Build history of the part. All positions in model axes, mm. A direction names the side the tool comes from. Round coordinates to 2 decimals unless told otherwise and drop trailing zeros. Order: outer loops, then holes, each group sorted by start corner. A loop starts at its lowest first (then second) coordinate and runs counter-clockwise, first axis right, second up. Notation, with made-up numbers: M 14.25,30 L 66.25,30 A18 ccw 66.25,45 Z; hole C 55,-17 d7. An arc over 180 degrees is marked long. Use CSV: the item, a comma, the result in double quotes.
from build123d import *

# Parameters (mm, degrees)
SKETCH3_R           = 43
SKETCH3_R_2         = 41
BOSS_EXTRUDE1_DEPTH = 200


with BuildPart() as part:
    # Sketch3 → Boss-Extrude1 (new body)
    with BuildSketch(Plane(origin=(0, 0, 0), x_dir=(1, 0, 0), z_dir=(0, 1, 0))):
        with BuildLine():
            Line((15.84339478, 39.974827602), (33, 43))
            Line((33, 43), (33, 54.159072389))
            Line((33, 54.159072389), (31, 54.159072389))
            Line((31, 54.159072389), (31, 45))
            Line((31, 45), (-31, 45))
            Line((-31, 45), (-31, 54))
            Line((-31, 54), (-33, 54))
            Line((-33, 54), (-33, 43))
            Line((-33, 43), (-15.84339478, 39.974827602))
            ThreePointArc((-15.84339478, 39.974827602), (0, 43), (15.84339478, 39.974827602))
        make_face()
        Circle(SKETCH3_R)
        Circle(SKETCH3_R_2, mode=Mode.SUBTRACT)
    extrude(amount=BOSS_EXTRUDE1_DEPTH)


solid = part.part
(1) Tool access for faces 1 (the face through (-9, 99, 40)), 2 (the face through (-33, 99, -49)), 3 (the face through (16, 0, -38)), 4 (the face through (31, 99, -50)), 5 (the face through (33, 99, -49)): list every direction of +Z, -Z, +X, -X, +Y, -Y with a clear straight run to the whole face (end or side of a thin tool).
Answer block:
face 1,"+Y, -Y"
face 2,"-Z, -X, +Y, -Y"
face 3,"+Z, -Z, +X, -X, -Y"
face 4,"-Z, +Y, -Y"
face 5,"-Z, +X, +Y, -Y"
(2) Cut at D-D, the plane x = 25. Give the cut face in (y, z), and give its area (3 significant figures).
Answer block:
outline,"M 0,-45 L 200,-45 L 200,-41.59 L 0,-41.59 Z; M 0,-34.99 L 200,-34.99 L 200,-32.5 L 0,-32.5 Z; M 0,32.5 L 200,32.5 L 200,34.99 L 0,34.99 Z"
area,"1,680 mm²"
(3) Cut at A-A, the plane x = 0. Give the cut face in (y, z), and give its area (3 significant figures).
Answer block:
outline,"M 0,-45 L 200,-45 L 200,-41 L 0,-41 Z; M 0,41 L 200,41 L 200,43 L 0,43 Z"
area,"1,200 mm²"
(4) Cut at B-B, the plane y = 157.5. Give the cut face in (x, z), and give its area (3 significant figures).
Answer block:
outline,"M -33,-54 L -31,-54 L -31,-45 L 31,-45 L 31,-54.16 L 33,-54.16 L 33,-43 L 15.84,-39.97 A43 ccw long -15.84,-39.97 L -33,-43 Z; hole C 0,0 d82"
area,"779 mm²"
(5) Drop flat-ended pins along their axis: pin 1 (1 mm diameter, centred on x = -32, y = 89.5, fed in from -Z); pin 2 (2 mm diameter, centred on x = -26, y = 84, fed in from -Z); pin 3 (2.5 mm diameter, centred on y = 120.5, z = -50, fed in from +X). Give the stop position or say it passes through.
Answer block:
pin 1,"stops at z = -54"
pin 2,"stops at z = -45"
pin 3,"stops at x = 33"
(6) Wall check: line 1 (X direction, y = 20.5, z = 1.5); line 2 (Z direction, x = 0, y = 77.5); line 3 (Z direction, x = -19, y = 18.5). Give the ranges that are in metal, low to high. Write a range as from..to.
Answer block:
line 1,"x = -42.97..-40.97, 40.97..42.97"
line 2,"z = -45..-41, 41..43"
line 3,"z = -45..-40.53, -38.57..-36.33, 36.33..38.57"
(7) Cut at C-C, the plane z = 0. Give the cut face in (x, y), and give its area (3 significant figures).
Answer block:
outline,"M -43,0 L -41,0 L -41,200 L -43,200 Z; M 41,0 L 43,0 L 43,200 L 41,200 Z"
area,"800 mm²"
(8) Two-plate mould, pull along Z, no slides. Class faces 6 (the face through (0, 99, -45)), 7 (the face through (-24.5, 98.6, -41.5)), 8 (the face through (16, 200, -38)): released by +Z, released by -Z, zero draft, split by the parting line, or undercut.
Answer block:
face 6,"released by -Z"
face 7,"undercut"
face 8,"zero draft"
